Drawing for the job (mm, zero at the part's lowest x, y, z). Give positions to 0.01 mm unless a question says otherwise; leave off trailing zeros. Order: outer loops, then holes, each group sorted by start corner. A loop starts at its lowest first (then second) coordinate and runs counter-clockwise, first axis right, second up. Notation, with made-up numbers: (69, 20.5) - (107, 20.5) arc R19 ccw to (107, 30.5) - close; hole circle Ø4 at (39.25, 66). An arc over 180 degrees is marked (long way). Write each question's results on one line, items separated by ' | '. Start each with the question number.
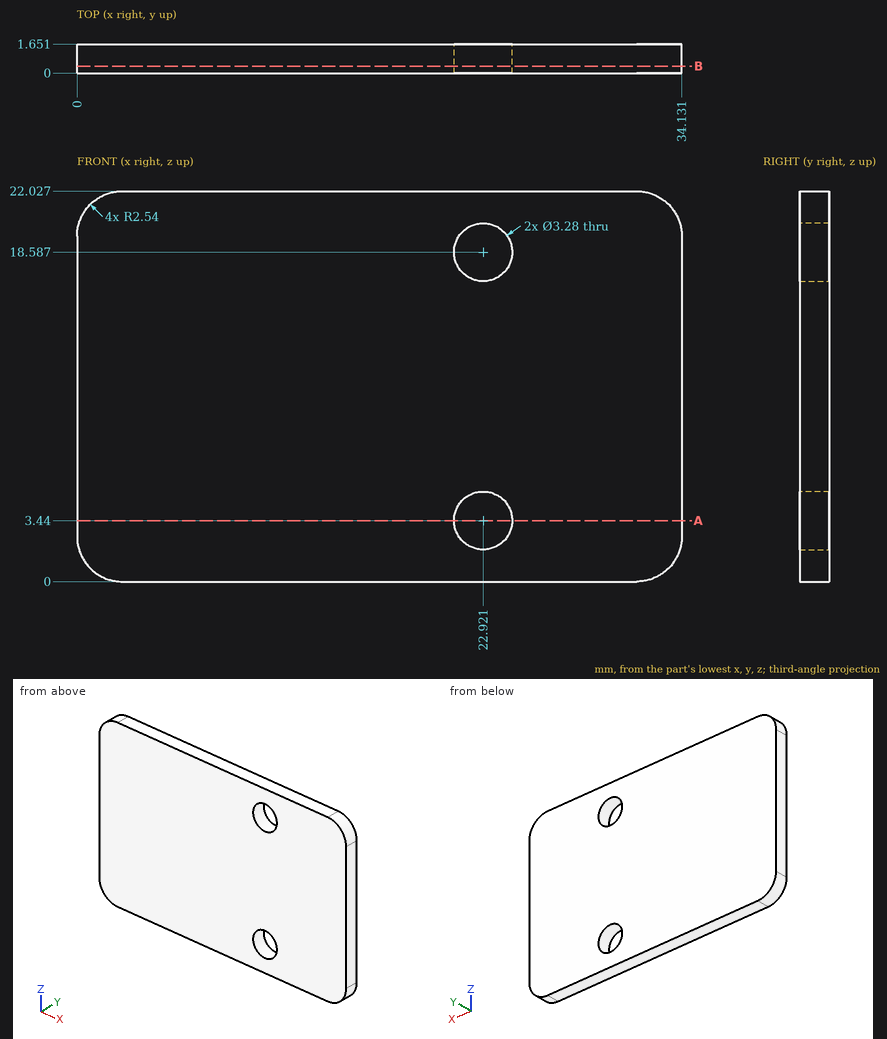
Item 1: Cut at A-A, the plane z = 3.44. List the corners of the cut face in (x, y).
Item 2: Probe line 1 along X through (y, z) = (1.2, 3.44); line 2 along X through (y, z) = (1.4, 19) (1 decimal); line 3 along X through (y, z) = (0.65, 1.5). List the from-to ranges inside material, lowest first. Write a range as from..to.
Item 3: Cut at B-B, the plane y = 0.4. List the corners of the cut face in (x, z), then the cut area to 3 significant figures.
Values found:
1) outline: (0, 0) - (21.28, 0) - (21.28, 1.65) - (0, 1.65) - close; (24.56, 0) - (34.13, 0) - (34.13, 1.65) - (24.56, 1.65) - close
2) line 1: x = 0..21.28, 24.56..34.13 | line 2: x = 0..21.3, 24.5..34.1 | line 3: x = 0.22..33.91
3) outline: (0, 2.54) arc R2.54 ccw to (2.54, 0) - (31.59, 0) arc R2.54 ccw to (34.13, 2.54) - (34.13, 19.49) arc R2.54 ccw to (31.59, 22.03) - (2.54, 22.03) arc R2.54 ccw to (0, 19.49) - close; hole circle Ø3.28 at (22.92, 3.44); hole circle Ø3.28 at (22.92, 18.59) | area: 729 mm2
